CAD build for the part. Positions are in the model's coordinates, mm. A direction names the side the tool comes from. Give positions to 0.01 mm unless a question says otherwise; leave off trailing zeros. Loops run counter-clockwise (first coordinate to the right, second up) from the corner with the lowest first, then second, coordinate; pieces in that order, holes last.
Item 1: Saw through at C-C on z = 1.5. Give the cut face in (x, y), plus the area to 3 significant figures.
Item 2: Saw through at D-D on y = 7. Give the cut face in (x, z).
Item 3: Saw through at B-B on y = -5. Give the cut face in (x, z).
Item 4: Which spindle directions (+Z, -Z, +X, -X, +Y, -Y) get a long thin tool onto all of the face, cutting with end or side? Do faces 4 (the flat face through (-8.479, 26.141, -6.614)), 5 (the flat face through (0, -5, -26.498)), 6 (the flat face through (0.098, 26.741, -20.347)), 7 (the flat face through (-8, 28, -14)). Say none if no direction does.
Item 5: Mould opens along X. For faces 1 (the flat face through (23, -5, 57)), 2 (the flat face through (-8.52, 26.74, -18.82)), 3 (the flat face through (0, -15, 5)) say: released by +X, released by -X, zero draft, split by the parting line, or undercut.
Item 6: Probe probe 1 along Y at (x, z) = (-8, 6); probe 2 along Y at (x, z) = (-3, 1); probe 3 along X at (y, z) = (6.5, 58). List the from-to ranges inside material, lowest first.
Item 7: Drop flat-ended pins along their axis: P1, Ø4, axis at y = 24, z = -13, coming from the -X side; P2, Ø13, axis at x = -0.5, y = 22, coming from the +Z side; P3, Ø6, axis at x = 1.5, z = 8.5, coming from the +Y side; P4, Ø8, axis at y = -6.5, z = 17.5, coming from the -X side. Give the stop position or say it passes through.
from build123d import *

# Parameters (mm, degrees)
BOSS_EXTRUDE1_DEPTH      = 25
BOSS_EXTRUDE1_DEPTH_BACK = 25
SKETCH1_R                = 25
BOSS_EXTRUDE4_DEPTH      = 20
BOSS_EXTRUDE4_DEPTH_BACK = 20
SKETCH9_W                = 85
SKETCH9_H                = 20
SHELL3_START             = -18
SHELL3_DEPTH             = 36
SHELL3_START_2           = -23
SHELL3_2_OUTLINE_R       = 23
SHELL3_2_DEPTH           = 46
FILLET2_R                = 5
BOSS_EXTRUDE5_DEPTH      = 10
BOSS_EXTRUDE5_DEPTH_BACK = 10
SKETCH5_W                = 40
SKETCH5_H                = 33.01510515
BOSS_EXTRUDE3_DEPTH      = 5
CUT_EXTRUDE2_REACH       = 111.266
SKETCH8_R                = 7.5
SKETCH12_W               = 16
SKETCH12_H               = 5.10776434
CUT_EXTRUDE3_DEPTH       = 119.899470043
CHAMFER2_SIZE            = 3
SKETCH13_R               = 15.5
CUT_EXTRUDE4_DEPTH       = 1


# Read off the part's stored shape, not the designer's step: Shell3
with BuildPart() as part:
    # Sketch1 → Boss-Extrude1 (new, two sides: drawn at the far end of the back side and taken through both)
    with BuildSketch(Plane(origin=(0, 0, 0), x_dir=(0, 0, -1), z_dir=(1, 0, 0)).offset(-BOSS_EXTRUDE1_DEPTH_BACK)):
        with Locations((-56.501901141, -5)):
            Circle(SKETCH1_R)
    extrude(amount=BOSS_EXTRUDE1_DEPTH + BOSS_EXTRUDE1_DEPTH_BACK)

    # Sketch9 → Boss-Extrude4 (add, two sides: drawn at the far end of the back side and taken through both)
    with BuildSketch(Plane(origin=(0, 0, 0), x_dir=(0, 0, -1), z_dir=(1, 0, 0)).offset(-BOSS_EXTRUDE4_DEPTH_BACK)):
        with Locations((-14.001901141, -5)):
            Rectangle(SKETCH9_W, SKETCH9_H)
    extrude(amount=BOSS_EXTRUDE4_DEPTH + BOSS_EXTRUDE4_DEPTH_BACK)

    # Shell3 outline → Shell3 (cut)
    with BuildSketch(Plane.YZ.offset(SHELL3_START)):
        with BuildLine():
            ThreePointArc((3, 34.938042488), (-5, 79.501901141), (-13, 34.938042488))
            Line((-13, 34.938042488), (-13, -26.498098859))
            Line((-13, -26.498098859), (3, -26.498098859))
            Line((3, -26.498098859), (3, 34.938042488))
        make_face()
    extrude(amount=SHELL3_DEPTH, mode=Mode.SUBTRACT)

    # Shell3 2 outline → Shell3 2 (cut)
    with BuildSketch(Plane.YZ.offset(SHELL3_START_2)):
        with Locations((-5, 56.501901141)):
            Circle(SHELL3_2_OUTLINE_R)
    extrude(amount=SHELL3_2_DEPTH, mode=Mode.SUBTRACT)

    # Fillet2
    fillet2_edges = [part.edges().sort_by_distance(p)[0] for p in [
        (0, 5, -28.498098859),
        (-20, -5, -28.498098859),
        (0, -15, -28.498098859),
        (20, -5, -28.498098859),
    ]]
    fillet(fillet2_edges, radius=FILLET2_R)

    # Sketch11 → Boss-Extrude5 (add, two sides: drawn at the far end of the back side and taken through both)
    with BuildSketch(Plane.ZY.offset(-BOSS_EXTRUDE5_DEPTH_BACK)):
        Polygon((-0.876282257, 5), (-9.456060259, 47.882592183), (-18.563824599, 47.882592183), (-22.259728969, 4.059726083), align=None)
    extrude(amount=BOSS_EXTRUDE5_DEPTH + BOSS_EXTRUDE5_DEPTH_BACK)

    # Sketch5 → Boss-Extrude3 (add)
    with BuildSketch(Plane(origin=(0, 47.882592183, 0), x_dir=(1, 0, 0), z_dir=(0, 1, 0))):
        with Locations((0, 9.154141988)):
            Rectangle(SKETCH5_W, SKETCH5_H)
    extrude(amount=BOSS_EXTRUDE3_DEPTH)

    # Sketch8 → Cut-Extrude2 (cut, up to next)
    with BuildSketch(Plane.ZY.offset(25), mode=Mode.PRIVATE) as cut_extrude2_sk1:
        with Locations((56.501901141, -5)):
            Circle(SKETCH8_R)
    cut_extrude2_tool1 = extrude(cut_extrude2_sk1.sketch, amount=-CUT_EXTRUDE2_REACH, mode=Mode.PRIVATE) & part.part
    add(cut_extrude2_tool1.solids().sort_by_distance((-25, -5, 56.501901))[0], mode=Mode.SUBTRACT)

    # Sketch12 → Cut-Extrude3 (cut, through all)
    with BuildSketch(Plane(origin=(0, 52.882592183, 0), x_dir=(1, 0, 0), z_dir=(0, 1, 0))):
        with Locations((0, 14.009942429)):
            Rectangle(SKETCH12_W, SKETCH12_H)
    extrude(amount=-CUT_EXTRUDE3_DEPTH, mode=Mode.SUBTRACT)

    # Chamfer2
    chamfer2_edges = [part.edges().sort_by_distance(p)[0] for p in [
        (10, 26.441296092, -20.372126679),
        (10, 26.441296092, -5.166171258),
        (-10, 26.441296092, -5.166171258),
        (-10, 26.441296092, -20.372126679),
    ]]
    chamfer(chamfer2_edges, length=CHAMFER2_SIZE)

    # Sketch13 → Cut-Extrude4 (cut)
    with BuildSketch(Plane(origin=(0, 52.882592183, 0), x_dir=(1, 0, 0), z_dir=(0, 1, 0))):
        with Locations(Location((0, 9.154141988, 0), (0, 0, 270))):
            Circle(SKETCH13_R)
    extrude(amount=-CUT_EXTRUDE4_DEPTH, mode=Mode.SUBTRACT)


solid = part.part
Results below:
1. outline: (-20, -15) - (20, -15) - (20, 5) - (-20, 5) - close; (-20, 47.88) - (20, 47.88) - (20, 52.88) - (11.26, 52.88) - (11.26, 51.88) - (-11.26, 51.88) - (-11.26, 52.88) - (-20, 52.88) - close; hole (-18, -13) - (18, -13) - (18, 3) - (-18, 3) - close
1. area: 401 mm2
2. outline: (-25, 34.57) - (25, 34.57) - (25, 78.43) - (-25, 78.43) - close; (-10, -19) - (-7, -22.01) - (7, -22.01) - (10, -19) - (10, -4.34) - (7, -1.28) - (-7, -1.28) - (-10, -4.34) - close; hole (-23, 36.88) - (23, 36.88) - (23, 76.12) - (-23, 76.12) - close; hole (-8, -16.56) - (8, -16.56) - (8, -11.46) - (-8, -11.46) - close
3. outline: (-25, 31.5) - (-20, 31.5) - (-20, -23.5) arc R5 ccw to (-15, -28.5) - (15, -28.5) arc R5 ccw to (20, -23.5) - (20, 31.5) - (25, 31.5) - (25, 81.5) - (-25, 81.5) - (-25, 64) - (-23, 64) - (-23, 79.5) - (23, 79.5) - (23, 33.5) - (18, 33.5) - (18, -26.5) - (-18, -26.5) - (-18, 33.5) - (-23, 33.5) - (-23, 49) - (-25, 49) - close
4. face 4: -X
4. face 5: none
4. face 6: -Z, +X, -X
4. face 7: +Y, -Y
5. face 1: undercut
5. face 2: released by -X
5. face 3: zero draft
6. probe 1: y = -15 to -13, 3 to 5, 47.88 to 52.88
6. probe 2: y = -15 to -13, 3 to 5, 47.88 to 51.88
6. probe 3: x = -25 to -23, 23 to 25
7. P1: stops at x = -10
7. P2: stops at z = 70.81
7. P3: stops at y = 52.88
7. P4: stops at x = -20
